Geometry check sheet. Reference: the model listing, model coordinates, mm. Round coordinates to 2 decimals unless told otherwise and drop trailing zeros. Order: outer loops, then holes, each group sorted by start corner. A loop starts at its lowest first (then second) coordinate and runs counter-clockwise, first axis right, second up.
(1) Material ranges on line 1 along Z through (x, y) = (-31, 6.75); line 2 along X through (y, z) = (2.25, -9.5); line 3 along Z through (x, y) = (16.5, 2.5), recorded low to high.
(2) Sectioned sample at B-B (z = -19). Record the boundary of the cut face in (x, y).
(3) Sectioned sample at A-A (x = 0). Record the boundary of the cut face in (y, z), plus the area to 3 significant figures.
(4) Sectioned sample at D-D (y = 6.5). Give the number of separate pieces and of enclosed holes in the cut face, plus the area to 3 significant figures.
(5) Go/stop test with flat-tipped pins: pin 1 (4.5 mm diameter, centred on x = -41, z = 0, fed in from -Y); pin 2 (8 mm diameter, centred on x = 41, z = 0, fed in from +Y); pin 3 (1 mm diameter, centred on y = 7.5, z = 25, fed in from +X). Record where each tip stops, or that it passes through.
(6) Sectioned sample at C-C (x = -53.5). Record the boundary of the cut face in (y, z).
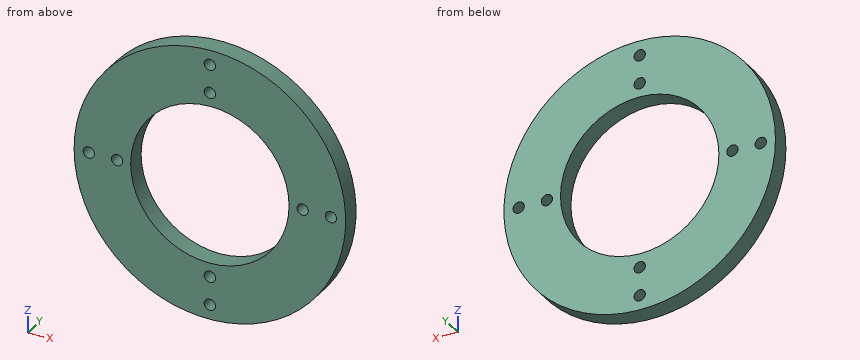
Autodesk Inventor part; units mm, degrees
ref_plane "YZ Plane" through (0, 0, 0) normal (1, 0, 0) x (0, 1, 0)
ref_plane "XZ Plane" through (0, 0, 0) normal (0, 1, 0) x (-1, 0, 0)
ref_plane "XY Plane" through (0, 0, 0) normal (0, 0, 1) x (1, 0, 0)
sketch "Sketch1" plane through (0, 0, 0) normal (0, 1, 0) x (-1, 0, 0)
  circle A0 centre (0, 0) radius 35
  circle A1 centre (0, 0) radius 60
  dimension "d0" = 70
  dimension "d1" = 120
extrude "Extrusion1" add sketch "Sketch1" along normal blind 8.5
sketch "Sketch2" plane through (0, 8.5, 0) normal (0, 1, 0) x (1, 0, 0)
  circle A0 centre (-41, 0) radius 2.5
  circle A1 centre (-53.5, 0) radius 2.5
  line L0 (-41, 0) -> (0, 0) construction
  line L1 (-41, 0) -> (-53.5, 0) construction
  dimension "d4" = 5
  dimension "d5" = 5
  dimension "d6" = 41
  dimension "d7" = 53.5
extrude "Extrusion2" cut sketch "Sketch2" against normal through all
pattern_circular "Circular Pattern1" count 4 over 360 about axis through (0, 0, 0) along (0, 1, 0) of "Extrusion2"
properties part number "Bearing" material "Aluminum 6061"
Answer below:
1. line 1: z = -51.37 to -16.25, 16.25 to 51.37
1. line 2: x = -59.24 to -33.69, 33.69 to 59.24
1. line 3: z = -57.69 to -30.87, 30.87 to 57.69
2. outline: (-56.91, 0) - (-29.39, 0) - (-29.39, 8.5) - (-56.91, 8.5) - close; (29.39, 0) - (56.91, 0) - (56.91, 8.5) - (29.39, 8.5) - close
3. outline: (0, -60) - (8.5, -60) - (8.5, -56) - (0, -56) - close; (0, -51) - (8.5, -51) - (8.5, -43.5) - (0, -43.5) - close; (0, -38.5) - (8.5, -38.5) - (8.5, -35) - (0, -35) - close; (0, 35) - (8.5, 35) - (8.5, 38.5) - (0, 38.5) - close; (0, 43.5) - (8.5, 43.5) - (8.5, 51) - (0, 51) - close; (0, 56) - (8.5, 56) - (8.5, 60) - (0, 60) - close
3. area: 255 mm2
4. separate pieces: 1
4. enclosed holes: 9
4. area: 7,300 mm2
5. pin 1: passes through
5. pin 2: stops at y = 8.5
5. pin 3: stops at x = 54.77
6. outline: (0, -27.16) - (8.5, -27.16) - (8.5, -2.5) - (0, -2.5) - close; (0, 2.5) - (8.5, 2.5) - (8.5, 27.16) - (0, 27.16) - close
